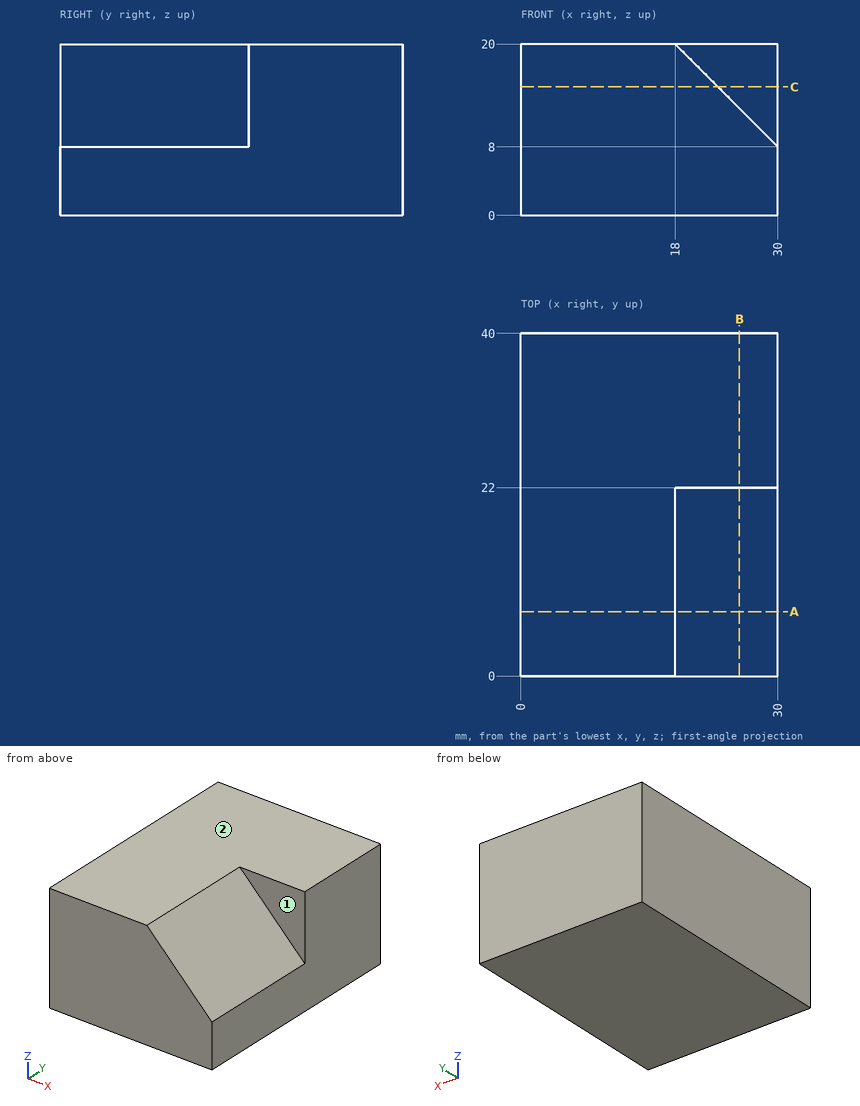
Source: three-view drawing plus pictorial views. Frame: mm from the lowest corner of the part. A direction names the side the tool comes from. Give positions to 0.01 mm unless a question says otherwise; leave off trailing zeros. Order: outer loops, then holes, each group sorted by start corner. A loop starts at its lowest first (then second) coordinate and runs counter-clockwise, first axis right, second up.
1. Section C-C on z = 15. Return the cut outline in (x, y), and give its area (3 significant figures).
Derived:
outline: (0, 0) - (23, 0) - (23, 22) - (30, 22) - (30, 40) - (0, 40) - close
area: 1,050 mm2
2. Section A-A on y = 7.5. Return the cut outline in (x, z).
Derived:
outline: (0, 0) - (30, 0) - (30, 8) - (18, 20) - (0, 20) - close
3. Reachability of the marked faces 1 and 2 from +Z, -Z, +X, -X, +Y, -Y: full face, straight path, thin tool, end or side. Return the list, or none.
Derived:
face 1: +Z, +X, -Y
face 2: +Z, +X, -X, +Y, -Y
4. Material intervals for L1, parallel to X at y = 4, z = 18; L2, parallel to Z at x = 23.5, y = 9; L3, parallel to Y at x = 28, z = 12, sorted ascending.
Derived:
L1: x = 0 to 20
L2: z = 0 to 14.5
L3: y = 22 to 40
5. Pin query (flat end, axial travel): pin 1 (1.5 mm diameter, centred on y = 11, z = 10, fed in from +X). Return the tip coordinate at first contact, or that it passes through.
Derived:
pin 1: stops at x = 28.75
6. Section B-B on x = 25.5. Return the cut outline in (y, z), and give its area (3 significant figures).
Derived:
outline: (0, 0) - (40, 0) - (40, 20) - (22, 20) - (22, 12.5) - (0, 12.5) - close
area: 635 mm2
